Source: three-view drawing plus pictorial views. Frame: mm from the lowest corner of the part. A direction names the side the tool comes from. Give positions to 0.01 mm unless a question says otherwise; leave off trailing zeros. Order: outer loops, then holes, each group sorted by start corner. A loop starts at its lowest first (then second) coordinate and runs counter-clockwise, first axis right, second up. Notation, with made-up numbers: (67, 45) -> (85, 45) arc R18 ccw to (85, 56) -> close; hole circle Ø6 at (-11.75, 8.5). An arc over 180 degrees is marked (long way). Write item = value, one per line.
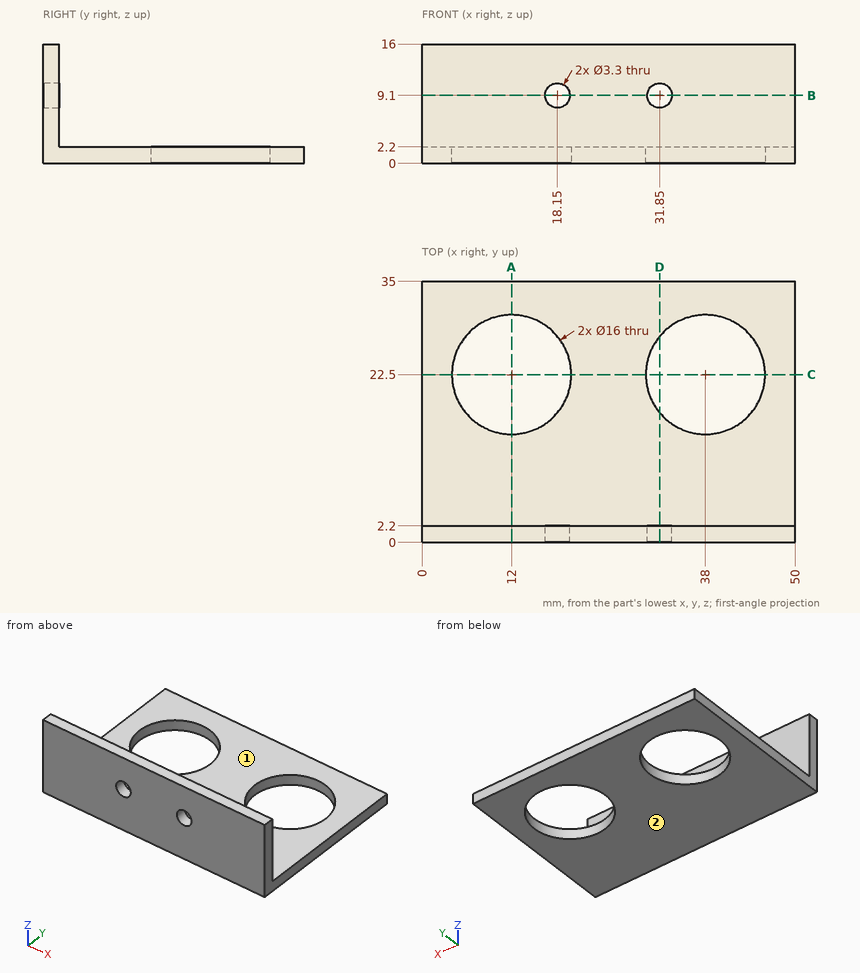
1) Section query A-A (x = 12). Output: boundary loops of the cut face in (y, z).
Check sheet entries:
outline = (0, 0) -> (14.5, 0) -> (14.5, 2.2) -> (2.2, 2.2) -> (2.2, 16) -> (0, 16) -> close; (30.5, 0) -> (35, 0) -> (35, 2.2) -> (30.5, 2.2) -> close
2) Section query D-D (x = 31.85). Output: boundary loops of the cut face in (y, z), plus the area to 3 significant figures.
Check sheet entries:
outline = (0, 0) -> (17.38, 0) -> (17.38, 2.2) -> (2.2, 2.2) -> (2.2, 7.45) -> (0, 7.45) -> close; (0, 10.75) -> (2.2, 10.75) -> (2.2, 16) -> (0, 16) -> close; (27.62, 0) -> (35, 0) -> (35, 2.2) -> (27.62, 2.2) -> close
area = 77.6 mm²
3) First-contact query: P1, Ø4.5, axis at x = 18.15, z = 9.1, coming from the +Y side; P2, Ø21, axis at x = 38, y = 22.5, coming from the -Z side; P3, Ø8, axis at x = 16.5, y = 29.5, coming from the +Z side. Flat tips, straight axial feed; report the tip coordinate or a pass-through.
Check sheet entries:
P1 = 2.2
P2 = 0
P3 = 2.2
4) Section query C-C (y = 22.5). Output: boundary loops of the cut face in (x, z).
Check sheet entries:
outline = (0, 0) -> (4, 0) -> (4, 2.2) -> (0, 2.2) -> close; (20, 0) -> (30, 0) -> (30, 2.2) -> (20, 2.2) -> close; (46, 0) -> (50, 0) -> (50, 2.2) -> (46, 2.2) -> close
5) Reachability of the marked faces 1 and 2 from +Z, -Z, +X, -X, +Y, -Y: full face, straight path, thin tool, end or side. Return the list, or none.
Check sheet entries:
face_1 = +Z, +X, -X, +Y
face_2 = -Z, +X, -X, +Y, -Y
6) Line query: line 1 (X direction, y = 0.8, z = 9.1); line 2 (Y direction, x = 12, z = 1.7); line 3 (Y direction, x = 8, z = 8.25). Output: solid intervals per line, ascending. Write a range as from..to.
Check sheet entries:
line_1 = 0..16.5, 19.8..30.2, 33.5..50
line_2 = 0..14.5, 30.5..35
line_3 = 0..2.2
7) Section query B-B (z = 9.1). Output: boundary loops of the cut face in (x, y), plus the area to 3 significant figures.
Check sheet entries:
outline = (0, 0) -> (16.5, 0) -> (16.5, 2.2) -> (0, 2.2) -> close; (19.8, 0) -> (30.2, 0) -> (30.2, 2.2) -> (19.8, 2.2) -> close; (33.5, 0) -> (50, 0) -> (50, 2.2) -> (33.5, 2.2) -> close
area = 95.5 mm²
